Job drawing, mm, ordinate dimensions from the low corner. One solid piece. A direction names the side the tool comes from. Round coordinates to 2 decimals unless told otherwise and drop trailing zeros. Answer as CSV lines item,"result". Start each with the question number.
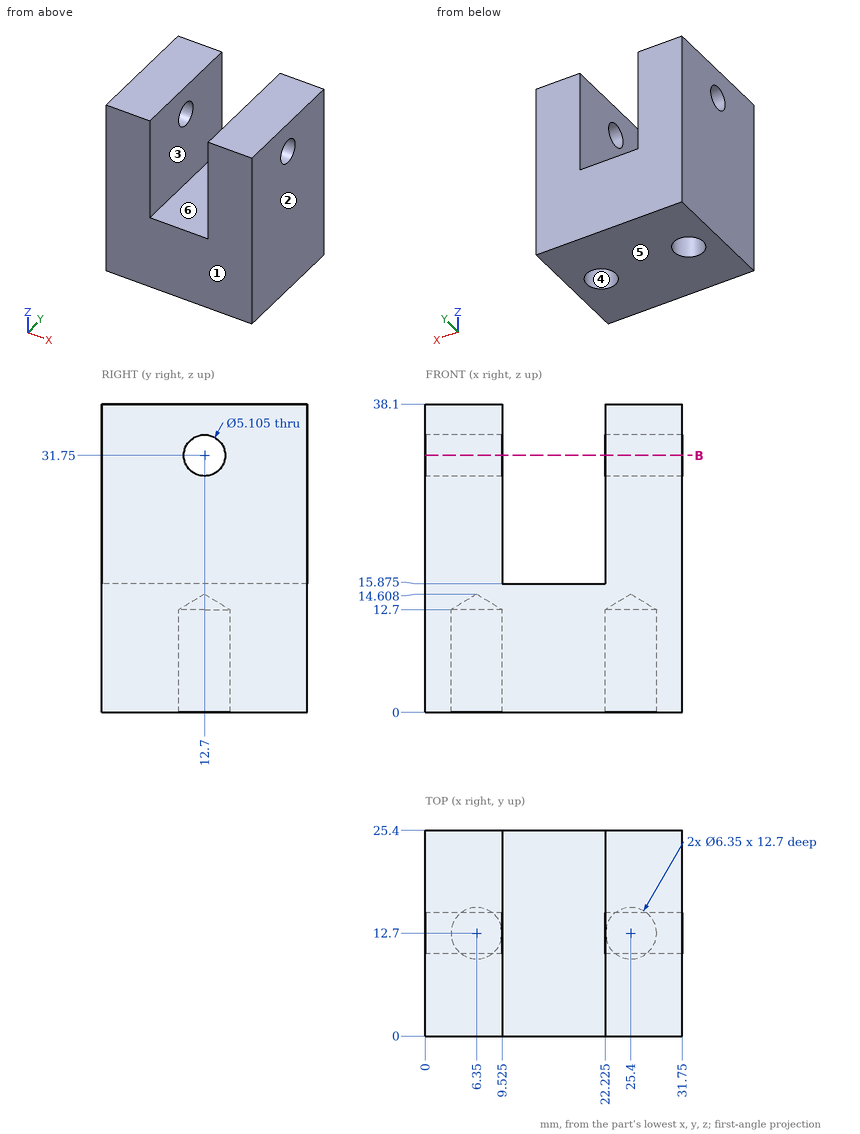
Q1. Band-saw the part on B-B, the plane z = 31.75. Give the number of separate pieces and of enclosed holes in the cut face.
Q2. Pin check, flat tips, straight feed: pin 1 Ø3 at (y, z) = (12.7, 31.75) entering from +X; pin 2 Ø10 at (x, y) = (16.5, 11) entering from +Z (3 decimals); pin 3 Ø5.5 at (x, y) = (25.4, 12.7) entering from -Z (1 decimal). Stop position of each tip, or through.
Q3. Two-plate mould, pull along X, no slides. Class the marked faces 1, 2 and 3: released by +X, released by -X, zero draft, split by the parting line, or undercut.
Q4. Wall check: probe 1 along Z at (x, y) = (16, 8.75) (1 decimal); probe 2 along Y at (x, z) = (6.35, 2.75) (1 decimal); probe 3 along Y at (x, z) = (4.5, 33.5). Give the ranges that are in metal, low to high. Write a range as [from, to].
Q5. Tool access for the marked faces 4, 5 and 6: list every direction of +Z, -Z, +X, -X, +Y, -Y with a clear straight run to the whole face (end or side of a thin tool).
Reported:
1,separate pieces,"4"
1,enclosed holes,"0"
2,pin 1,"passes through"
2,pin 2,"stops at z = 15.875"
2,pin 3,"stops at z = 13"
3,face 1,"zero draft"
3,face 2,"released by +X"
3,face 3,"undercut"
4,probe 1,"z = [0, 15.9]"
4,probe 2,"y = [0, 9.5], [15.9, 25.4]"
4,probe 3,"y = [0, 10.84], [14.56, 25.4]"
5,face 4,"-Z"
5,face 5,"-Z, +X, -X, +Y, -Y"
5,face 6,"+Z, +Y, -Y"
